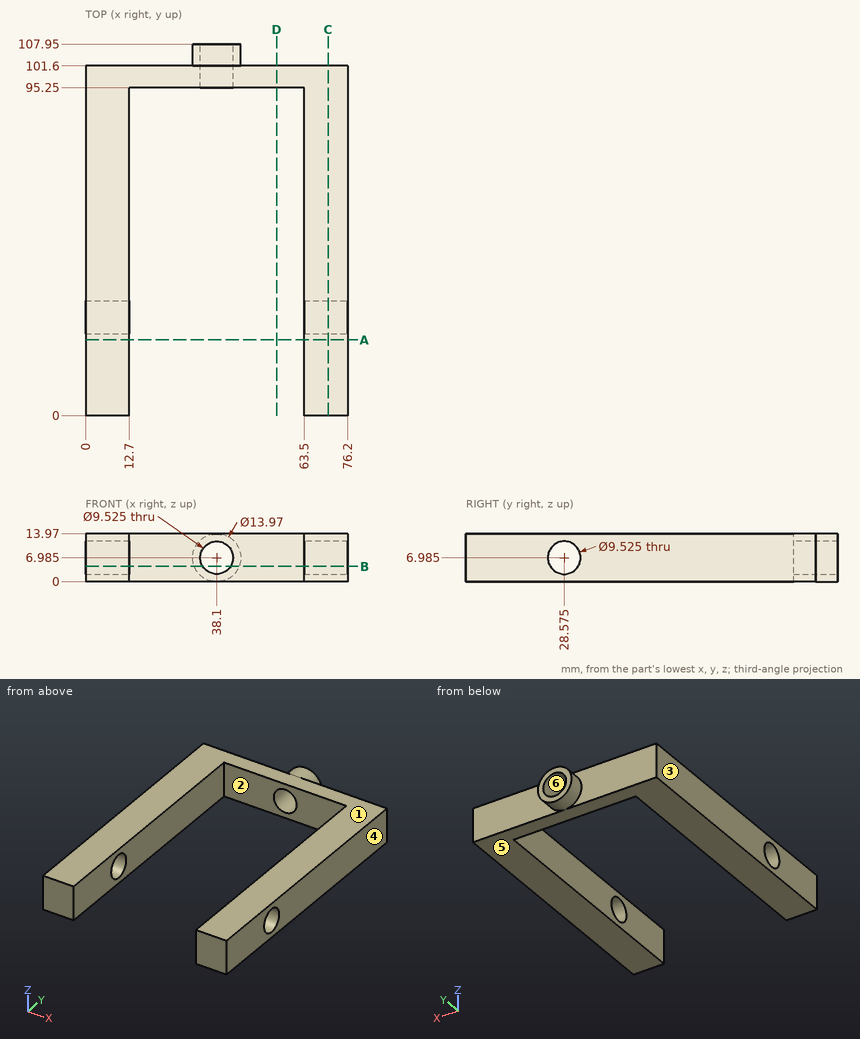
For this review, use the dimensioned drawing (mm, ordinates from the lowest corner) and the shaded views. A direction names the side the tool comes from. Coordinates: 2 decimals unless noted, no trailing zeros. Loops run counter-clockwise (first coordinate to the right, second up) from the corner with the lowest first, then second, coordinate; pieces in that order, holes last. Notation, with made-up numbers: (-39.5, 78.25) -> (-12.5, 78.25) arc R25 cw to (-12.5, 92.25) -> close; hole circle Ø5 at (57, -38). An arc over 180 degrees is marked (long way). Use a Markdown table: item, result. Add a question column.
1. Clearance check with flat-ended pins moving along their axes: pin 1 Ø4 at (x, z) = (55.5, 7) entering from -Y; pin 2 Ø5.5 at (y, z) = (28.575, 6.985) entering from -X; pin 3 Ø7 at (x, z) = (26.5, 4.5) entering from +Y. State where each tip first meets the part, or that it passes through.
2. Add section D-D on x = 55.5. Write out the cut boundary in (y, z).
3. Draft analysis for pull direction X (two halves, no side actions). For the marked faces 3, 4, 5 and 6, state which applies: pulls with the +X half, pulls with the -X half, needs draft (parallel to the pull), parting line crosses it, or undercut.
4. Add section C-C on x = 70.5. Write out the cut boundary in (y, z) (1 decimal), plus the area to 3 significant figures.
5. Machinability: for the marked faces 1 and 2, which of the approach directions +Z, -Z, +X, -X, +Y, -Y give a long, thin tool a straight path to every point of the face, cutting with its end or side? Answer none if there is none.
6. Add section B-B on z = 4.5. Write out the cut boundary in (x, y), plus the area to 3 significant figures.
7. To check wall thickness, follow line 1 (X direction, y = 88.5, z = 10.75); line 2 (Y direction, x = 20.5, z = 3.75); line 3 (Y direction, x = 32.5, z = 7.5). State the ranges of each line that lie inside material, in increasing order.
8. Add section A-A on y = 22. Write out the cut boundary in (x, z), plus the area to 3 significant figures.
Returned:
| question | item | result |
|---|---|---|
| 1 | pin 1 | stops at y = 95.25 |
| 1 | pin 2 | passes through |
| 1 | pin 3 | stops at y = 101.6 |
| 2 | outline | (95.25, 0) -> (101.6, 0) -> (101.6, 13.97) -> (95.25, 13.97) -> close |
| 3 | face 3 | pulls with the -X half |
| 3 | face 4 | pulls with the +X half |
| 3 | face 5 | needs draft |
| 3 | face 6 | undercut |
| 4 | outline | (0, 0) -> (101.6, 0) -> (101.6, 14) -> (0, 14) -> close; hole circle Ø9.5 at (28.6, 7) |
| 4 | area | 1,350 mm² |
| 5 | face 1 | +Z, +X, -X, +Y, -Y |
| 5 | face 2 | +Z, -Z, -Y |
| 6 | outline | (0, 0) -> (12.7, 0) -> (12.7, 24.51) -> (0, 24.51) -> close; (0, 32.64) -> (12.7, 32.64) -> (12.7, 95.25) -> (34.04, 95.25) -> (34.04, 107.95) -> (31.57, 107.95) -> (31.57, 101.6) -> (0, 101.6) -> close; (42.16, 95.25) -> (63.5, 95.25) -> (63.5, 32.64) -> (76.2, 32.64) -> (76.2, 101.6) -> (44.63, 101.6) -> (44.63, 107.95) -> (42.16, 107.95) -> close; (63.5, 0) -> (76.2, 0) -> (76.2, 24.51) -> (63.5, 24.51) -> close |
| 6 | area | 2,680 mm² |
| 7 | line 1 | x = 0 to 12.7, 63.5 to 76.2 |
| 7 | line 2 | y = 95.25 to 101.6 |
| 7 | line 3 | y = 95.25 to 107.95 |
| 8 | outline | (0, 0) -> (12.7, 0) -> (12.7, 13.97) -> (0, 13.97) -> close; (63.5, 0) -> (76.2, 0) -> (76.2, 13.97) -> (63.5, 13.97) -> close |
| 8 | area | 355 mm² |
